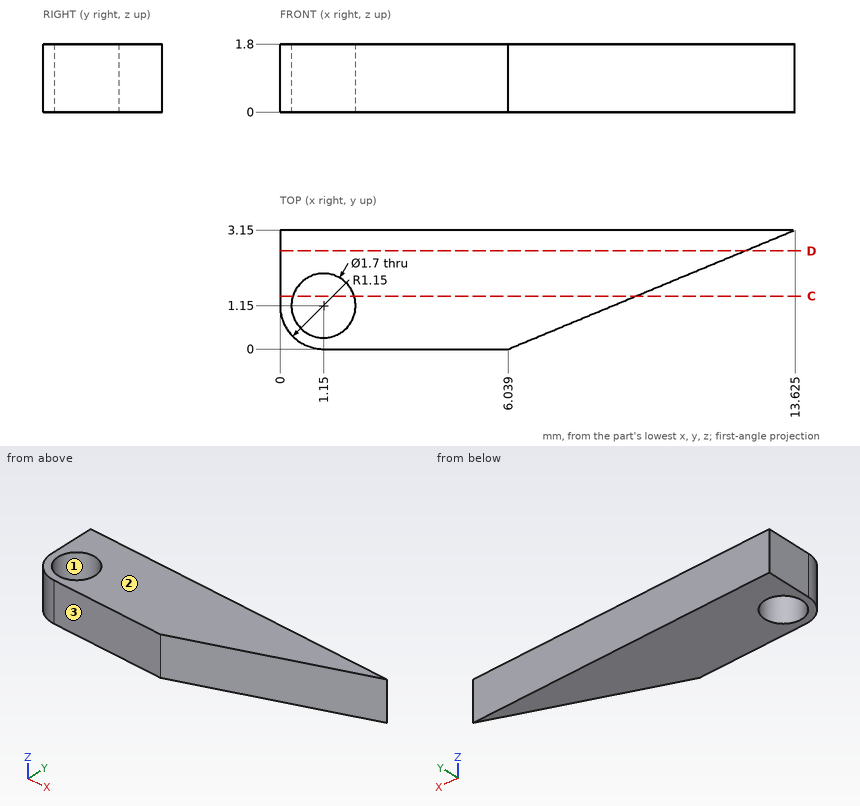
For this review, use the dimensioned drawing (mm, ordinates from the lowest corner) and the shaded views. Give positions to 0.01 mm unless a question says otherwise; leave off trailing zeros. Order: outer loops, then holes, each group sorted by start corner. A loop starts at its lowest first (then second) coordinate and runs counter-clockwise, first axis right, second up. Notation, with made-up numbers: (63.5, 53) -> (117.5, 53) arc R24 ccw to (117.5, 71) -> close; hole circle Ø6 at (-24, -7.5). An arc over 180 degrees is marked (long way). Write item = value, one per line. Start each with the question number.
(1) For L1, parallel to X at y = 1.65, z = 0.6 (1 decimal); L2, parallel to X at y = 1.2, z = 0.3 (1 decimal); L3, parallel to Y at x = 10.5, z = 0.7, list the stretches that pass through material, from the lowest coordinate up. Write a range as from..to.
(2) Take a section at D-D (y = 2.6). Write out the cut boundary in (x, z).
(3) Draft analysis for pull direction Y (two halves, no side actions). For the marked faces 1, 2 and 3, state which applies: +Y half, -Y half, draft (parallel to the pull), parting line (faces both ways), or undercut.
(4) Take a section at C-C (y = 1.4). Write out the cut boundary in (x, z).
Returned:
q1.L1 = 0..0.5, 1.8..10
q1.L2 = 0..0.3, 2..8.9
q1.L3 = 1.85..3.15
q2.outline = (0, 0) -> (12.3, 0) -> (12.3, 1.8) -> (0, 1.8) -> close
q3.face_1 = undercut
q3.face_2 = draft
q3.face_3 = -Y half
q4.outline = (0, 0) -> (0.34, 0) -> (0.34, 1.8) -> (0, 1.8) -> close; (1.96, 0) -> (9.41, 0) -> (9.41, 1.8) -> (1.96, 1.8) -> close
